from build123d import *

# Parameters (mm, degrees)
SKETCH1_R           = 16
SKETCH1_R_2         = 2.5
BOSS_EXTRUDE1_DEPTH = 6.5
SKETCH2_R           = 1.5
CUT_EXTRUDE1_DEPTH  = 24.542514734
SKETCH4_R           = 4.75
SKETCH4_R_2         = 2.5
BOSS_EXTRUDE2_DEPTH = 1
SKETCH5_R           = 4
SKETCH5_R_2         = 2.5
BOSS_EXTRUDE3_DEPTH = 7


with BuildPart() as part:
    # Sketch1 → Boss-Extrude1 (new body)
    with BuildSketch(Plane(origin=(0, 0, 0), x_dir=(0, 0, -1), z_dir=(1, 0, 0))):
        with Locations(Location((0, 0, 0), (0, 0, 180))):
            Circle(SKETCH1_R)
        with Locations(Location((0, 0, 0), (0, 0, 180))):
            Circle(SKETCH1_R_2, mode=Mode.SUBTRACT)
    extrude(amount=BOSS_EXTRUDE1_DEPTH)

    # Sketch2 → Cut-Extrude1 (cut, through all)
    with BuildSketch(Plane(origin=(6.5, 0, 0), x_dir=(0, 0, -1), z_dir=(1, 0, 0))):
        with Locations((0, 13)):
            Circle(SKETCH2_R)
        with Locations((13, 0)):
            Circle(SKETCH2_R)
        with Locations((0, -13)):
            Circle(SKETCH2_R)
        with Locations((-13, 0)):
            Circle(SKETCH2_R)
    extrude(amount=-CUT_EXTRUDE1_DEPTH, mode=Mode.SUBTRACT)

    # Sketch4 → Boss-Extrude2 (add)
    with BuildSketch(Plane(origin=(6.5, 0, 0), x_dir=(0, 0, -1), z_dir=(1, 0, 0))):
        Circle(SKETCH4_R)
        with Locations(Location((0, 0, 0), (0, 0, 180))):
            Circle(SKETCH4_R_2, mode=Mode.SUBTRACT)
    extrude(amount=BOSS_EXTRUDE2_DEPTH)

    # Sketch5 → Boss-Extrude3 (add)
    with BuildSketch(Plane(origin=(7.5, 0, 0), x_dir=(0, 0, -1), z_dir=(1, 0, 0))):
        Circle(SKETCH5_R)
        with Locations(Location((0, 0, 0), (0, 0, 180))):
            Circle(SKETCH5_R_2, mode=Mode.SUBTRACT)
    extrude(amount=BOSS_EXTRUDE3_DEPTH)


solid = part.part
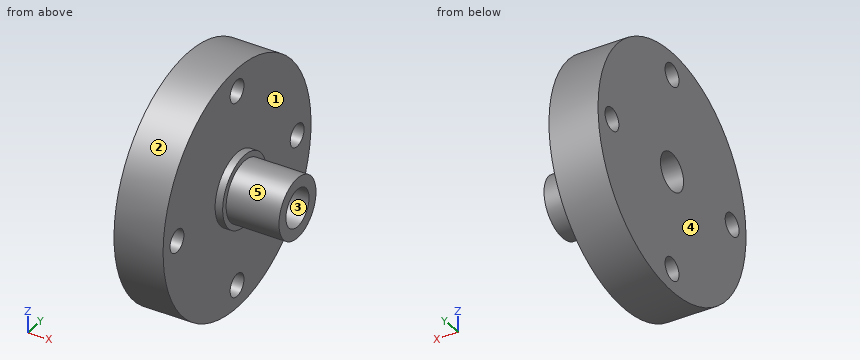
Check sheet for the modelled part. Datum: model origin and axes. Units: mm. Face numbers are marked on the shaded views. A direction names the side the tool comes from. Give positions to 0.01 mm unless a question says otherwise; leave off trailing zeros. Loops run counter-clockwise (first coordinate to the right, second up) from the corner with the lowest first, then second, coordinate; pieces in that order, holes last. Notation, with made-up numbers: M 38,18.25 L 61,18.25 A25 ccw 61,51.25 Z; hole C 80,77.25 d7. An arc over 180 degrees is marked long. Answer as a JSON object with one key per item and string values. Group by question number.
Q1. Access from +Z, -Z, +X, -X, +Y, -Y to the whole of each face (thin tool, end or side, straight path). Record for the marked faces 4 and 5.
Q2. Cross-section at D-D on x = 12.75. Record the cut outline in (y, z), then the cut area to 3 significant figures.
Q3. Cross-section at A-A on z = 0. Record the cut outline in (x, y), then the cut area to 3 significant figures.
Q4. Cross-section at C-C on y = -13. Record the cut outline in (x, z), then the cut area to 3 significant figures.
Q5. Go/stop test with flat-tipped pins: P1, Ø5, axis at y = -0.5, z = -1.5, coming from the +X side; P2, Ø2.5, axis at y = 0, z = -13, coming from the -X side; P3, Ø1.5, axis at x = 4, z = -5, coming from the +Y side; P4, Ø3, axis at x = 6, z = -7.5, coming from the +Y side. Record where each tip stops, or that it passes through.
Q6. Material ranges on line 1 along Y through (x, z) = (5.25, 0); line 2 along Z through (x, y) = (4, -1); line 3 along Y through (x, z) = (10.5, 0), recorded low to high. Write a range as [from, to].
Q7. Release check for a two-part mould opening along Z. For the marked faces 1, 2 and 3 record: released by +Z, released by -Z, zero draft, split by the parting line, or undercut.
Q8. Cross-section at B-B on x = 1.5. Record the cut outline in (y, z), then the cut area to 3 significant figures.
Evaluation:
{
 "1": {"face 4": "+Z, -Z, -X, +Y, -Y", "face 5": "+X"},
 "2": {"outline": "C 0,0 d8; hole C 0,0 d5", "area": "30.6 mm2"},
 "3": {"outline": "M 0,-16 L 6.5,-16 L 6.5,-14.5 L 0,-14.5 Z; M 0,-11.5 L 6.5,-11.5 L 6.5,-4.75 L 7.5,-4.75 L 7.5,-4 L 14.5,-4 L 14.5,-2.5 L 0,-2.5 Z; M 0,2.5 L 14.5,2.5 L 14.5,4 L 7.5,4 L 7.5,4.75 L 6.5,4.75 L 6.5,11.5 L 0,11.5 Z; M 0,14.5 L 6.5,14.5 L 6.5,16 L 0,16 Z", "area": "162 mm2"},
 "4": {"outline": "M 0,-9.33 L 6.5,-9.33 L 6.5,-1.5 L 0,-1.5 Z; M 0,1.5 L 6.5,1.5 L 6.5,9.33 L 0,9.33 Z", "area": "102 mm2"},
 "5": {"P1": "stops at x = 14.5", "P2": "passes through", "P3": "stops at y = 15.43", "P4": "stops at y = 14.83"},
 "6": {"line 1": "y = [-16, -14.5], [-11.5, -2.5], [2.5, 11.5], [14.5, 16]", "line 2": "z = [-15.97, -14.12], [-11.88, -2.29], [2.29, 11.88], [14.12, 15.97]", "line 3": "y = [-4, -2.5], [2.5, 4]"},
 "7": {"face 1": "zero draft", "face 2": "split by the parting line", "face 3": "undercut"},
 "8": {"outline": "C 0,0 d32; hole C -13,0 d3; hole C 0,0 d5; hole C 0,-13 d3; hole C 0,13 d3; hole C 13,0 d3", "area": "756 mm2"}
}
